Answer from the drawing. Dimensions are ordinates in mm from the lowest x, y and z of the part. A direction names the side the tool comes from. Give positions to 0.01 mm unless a question says otherwise; leave off trailing zeros. Loops run counter-clockwise (first coordinate to the right, second up) from the corner with the lowest first, then second, coordinate; pieces in that order, holes last. Notation, with made-up numbers: (-1, 11) -> (39, 11) arc R31 cw to (39, 40) -> close; hole circle Ø7 at (25, 35). An arc over 180 degrees is marked (long way). Write each question's results on one line, items separated by ' | '. Start each with the question number.
Item 1: Section B-B on x = 30 is taken. Write down the section's boundary in (y, z).
Item 2: Section C-C on x = 52.5 is taken. Write down the section's boundary in (y, z), and give its area (3 significant figures).
Item 3: Which of the six approach directions +Z, -Z, +X, -X, +Y, -Y give full straight-line access (tool end or side, diameter ignored) to the marked faces 1, 2, 3 and 4?
Item 4: Find the intervals of material crossed by line 1 (Z direction, x = 19, y = 7); line 2 (Y direction, x = 51.5, z = 72); line 3 (Z direction, x = 53.5, y = 8.5), in increasing order.
Item 5: Each of these flat-tipped pins is pushed along its axis until it touches: P1, Ø15, axis at y = 32.5, z = 66.5, coming from the -X side; P2, Ø4, axis at x = 33.5, z = 43.5, coming from the -Y side; P3, Ø6, axis at x = 18.5, z = 13.5, coming from the +Y side. Where does it stop, or does it pass through?
Item 6: Section A-A on y = 54 is taken. Write down the section's boundary in (x, z), and give its area (3 significant figures).
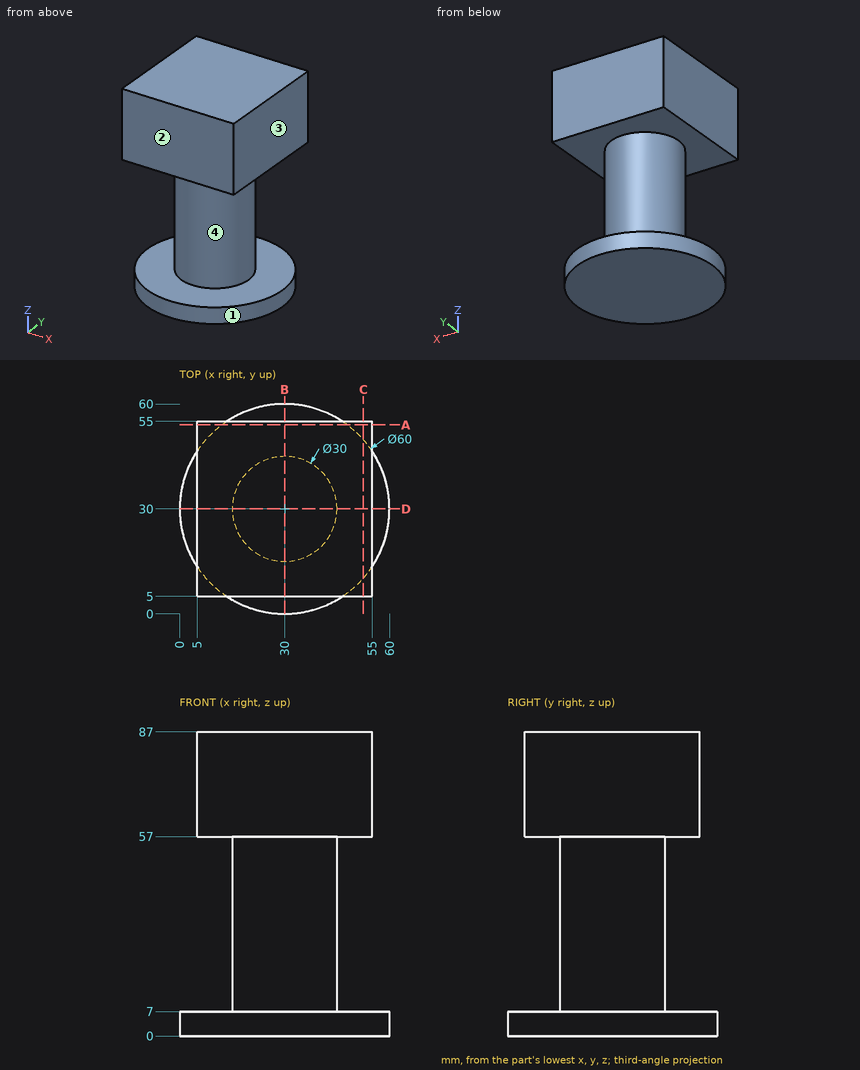
Findings:
1) outline: (0, 0) -> (60, 0) -> (60, 7) -> (45, 7) -> (45, 57) -> (55, 57) -> (55, 87) -> (5, 87) -> (5, 57) -> (15, 57) -> (15, 7) -> (0, 7) -> close
2) outline: (5, 57) -> (55, 57) -> (55, 87) -> (5, 87) -> close; (10.16, 0) -> (49.84, 0) -> (49.84, 7) -> (10.16, 7) -> close | area: 1,780 mm2
3) face 1: -Z | face 2: +Z, +X, -X, -Y | face 3: +Z, +X, +Y, -Y | face 4: none
4) line 1: 0 to 7, 57 to 87 | line 2: 5 to 55 | line 3: 57 to 87
5) P1: x = 5 | P2: y = 15.08 | P3: y = 42.36
6) outline: (5, 57) -> (55, 57) -> (55, 87) -> (5, 87) -> close; (12, 0) -> (48, 0) -> (48, 7) -> (12, 7) -> close | area: 1,750 mm2
